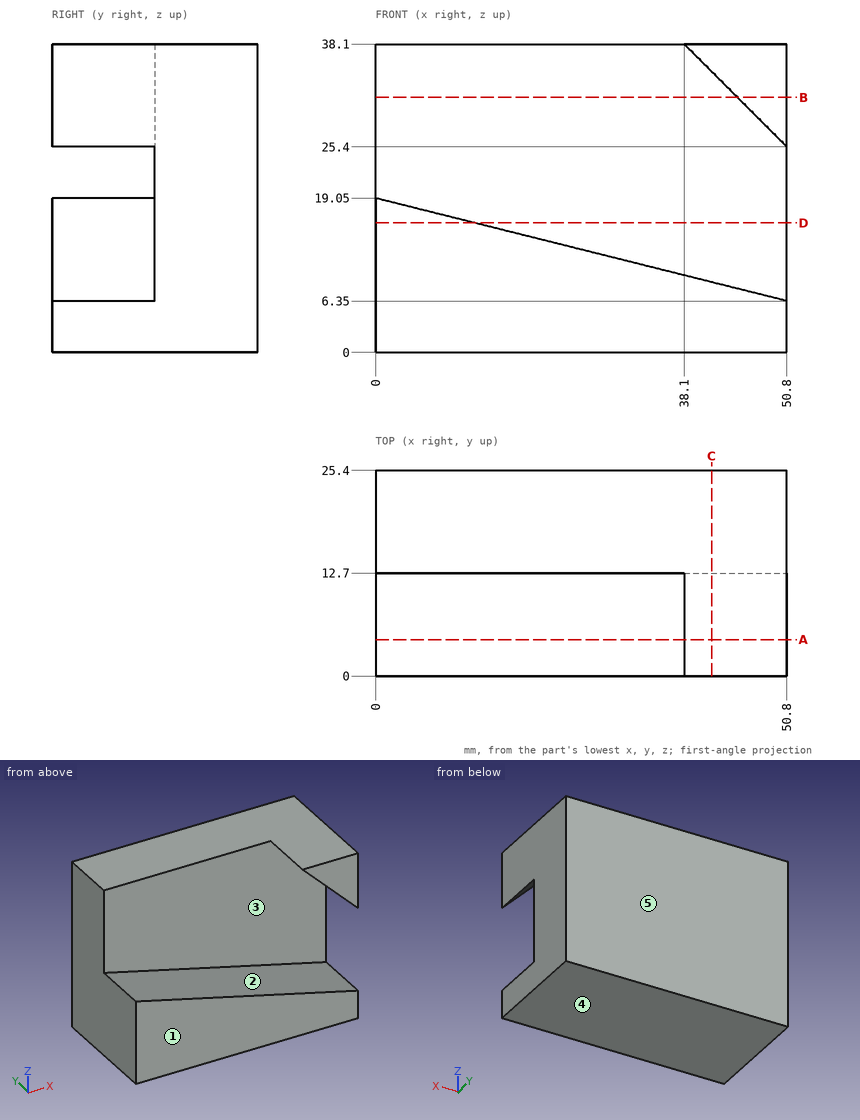
Can you work these out from the drawing? Everything is in mm from the part's minimum corner. A direction names the side the tool comes from. Coordinates: 2 decimals unless noted, no trailing zeros. Loops run counter-clockwise (first coordinate to the right, second up) from the corner with the lowest first, then second, coordinate; pieces in that order, holes last.
1) Which directions (+Z, -Z, +X, -X, +Y, -Y) give clear straight access to the entire face, cutting with the end or side of a thin tool? Please do the marked faces 1 and 2.
2) Thinking about a two-plate mould opening in Z: for the marked faces 3, 4 and 5, which applies, pulls with the +Z half, pulls with the -Z half, needs draft (parallel to the pull), parting line crosses it, or undercut?
3) Imagine slicing it at D-D on z = 16. List the corners of the cut face in (x, y) for me, plus the area to 3 significant figures.
4) For pin 1 (2 mm diameter, centred on x = 16.5, y = 4.5, fed in from +Z) (3 decimals), with a flat end and sliding along its axis, tell me the tip position at first contact or that it passes through.
5) Imagine slicing it at C-C on x = 41.5. List the corners of the cut face in (y, z) for me (3 decimals), plus the area to 3 significant figures.
6) I need wall thicknesses on probe 1 along Y at (x, z) = (14, 36.5); probe 2 along Z at (x, y) = (39, 5); probe 3 along X at (y, z) = (5, 31.5). Which ranges of each line are inside material? Lowest first, please.
7) Imagine slicing it at A-A on y = 4.5. List the corners of the cut face in (x, z) for me.
8) Imagine slicing it at B-B on z = 31.5. List the corners of the cut face in (x, y) for me.
Completed:
1. face 1: +Z, -Z, +X, -X, -Y
1. face 2: +X, -Y
2. face 3: undercut
2. face 4: pulls with the -Z half
2. face 5: needs draft
3. outline: (0, 0) - (12.2, 0) - (12.2, 12.7) - (50.8, 12.7) - (50.8, 25.4) - (0, 25.4) - close
3. area: 800 mm2
4. pin 1: stops at z = 15.175
5. outline: (0, 0) - (25.4, 0) - (25.4, 38.1) - (0, 38.1) - (0, 34.7) - (12.7, 34.7) - (12.7, 8.675) - (0, 8.675) - close
5. area: 637 mm2
6. probe 1: y = 12.7 to 25.4
6. probe 2: z = 0 to 9.3, 37.2 to 38.1
6. probe 3: x = 44.7 to 50.8
7. outline: (0, 0) - (50.8, 0) - (50.8, 6.35) - (0, 19.05) - close; (38.1, 38.1) - (50.8, 25.4) - (50.8, 38.1) - close
8. outline: (0, 12.7) - (44.7, 12.7) - (44.7, 0) - (50.8, 0) - (50.8, 25.4) - (0, 25.4) - close
